from build123d import *

# Parameters (mm, degrees)
SKETCH_1_W          = 10
SKETCH_1_H          = 10
SKETCH_1_W_2        = 8
SKETCH_1_H_2        = 8
EXTRUDE_1_DEPTH     = 50
SKETCH_2_R          = 3
SKETCH_2_R_2        = 1.6
CUT_EXTRUDE_1_DEPTH = 52.961524227
CUT_EXTRUDE_2_REACH = 53.962
SKETCH_4_R          = 2.6
SKETCH_6_R          = 1.6
CUT_EXTRUDE_4_DEPTH = 52.961524227


with BuildPart() as part:
    # ｽｹｯﾁ1 → 押し出し-薄板1 (new body)
    with BuildSketch(Plane.XY):
        with Locations((5, 5)):
            Rectangle(SKETCH_1_W, SKETCH_1_H)
        with Locations((5, 5)):
            Rectangle(SKETCH_1_W_2, SKETCH_1_H_2, mode=Mode.SUBTRACT)
    extrude(amount=EXTRUDE_1_DEPTH)

    # ｽｹｯﾁ2 → ｶｯﾄ - 押し出し1 (cut, through all)
    with BuildSketch(Plane(origin=(0, 10, 0), x_dir=(1, 0, 0), z_dir=(0, 1, 0))):
        with Locations(Location((5, -10.5, 0), (0, 0, 270))):
            Circle(SKETCH_2_R)
        with Locations(Location((5, -19.5, 0), (0, 0, 270))):
            Circle(SKETCH_2_R_2)
        with Locations(Location((5, -34.5, 0), (0, 0, 270))):
            Circle(SKETCH_2_R_2)
    extrude(amount=-CUT_EXTRUDE_1_DEPTH, mode=Mode.SUBTRACT)

    # ｽｹｯﾁ4 → ｶｯﾄ - 押し出し2 (cut, up to next)
    with BuildSketch(Plane.XZ, mode=Mode.PRIVATE) as cut_extrude_2_sk1:
        with Locations(Location((5, 19.5, 0), (0, 0, 270))):
            Circle(SKETCH_4_R)
    cut_extrude_2_tool1 = extrude(cut_extrude_2_sk1.sketch, amount=-CUT_EXTRUDE_2_REACH, mode=Mode.PRIVATE) & part.part
    add(cut_extrude_2_tool1.solids().sort_by_distance((5, 0, 19.5))[0], mode=Mode.SUBTRACT)

    # ｽｹｯﾁ6 → ｶｯﾄ - 押し出し4 (cut, through all)
    with BuildSketch(Plane(origin=(10, 0, 0), x_dir=(0, 0, -1), z_dir=(1, 0, 0))):
        with Locations(Location((-45, 5, 0), (0, 0, 90))):
            Circle(SKETCH_6_R)
    extrude(amount=-CUT_EXTRUDE_4_DEPTH, mode=Mode.SUBTRACT)


solid = part.part
Verification items for the finished model (mm, model axes). A direction names the side the tool comes from. Give positions to 0.01 mm unless a question says otherwise; leave off trailing zeros. Order: outer loops, then holes, each group sorted by start corner. A loop starts at its lowest first (then second) coordinate and runs counter-clockwise, first axis right, second up. Notation, with made-up numbers: M 19,89 L 27,89 A10 ccw 27,105 Z; hole C -31,28.25 d11. An arc over 180 degrees is marked long. Use one line per item in the form item = value. Start each with the question number.
Q1. Section check A-A (y = 2.75). Enter the section's corners in (x, z).
Q2. Section check D-D (z = 37.5). Enter the section's corners in (x, y).
Q3. Mould release check, pull along X, two halves, no side actions. Record for faces 1 (the flat face through (0.5, 5.1, 50)), 2 (the flat face through (10, 5, 25)), 3 (the flat face through (5, 9, 25)): +X half, -X half, draft (parallel to the pull), parting line (faces both ways), or undercut.
Q4. Section check B-B (z = 19.5). Enter the section's corners in (x, y), then the cut area to 3 significant figures.
Q5. Access from +Z, -Z, +X, -X, +Y, -Y to the whole of each face (thin tool, end or side, straight path). Record for faces 4 (the flat face through (5, 0, 25)), 5 (the flat face through (9, 5, 25)), 6 (the cylindrical face through (5.78, 0.49, 17.02)).
Q6. Scan lines: line 1 along X through (y, z) = (3.25, 3.5); line 2 along Z through (x, y) = (9.5, 5). Record each from-to range of solid material in increasing order. Write a range as [from, to].
Q7. Section check C-C (y = 5). Enter the section's corners in (x, z).
Evaluation:
q1.outline = M 0,0 L 1,0 L 1,50 L 0,50 Z; M 9,0 L 10,0 L 10,50 L 9,50 Z
q2.outline = M 0,0 L 10,0 L 10,10 L 0,10 Z; hole M 1,1 L 9,1 L 9,9 L 1,9 Z
q3.face_1 = draft
q3.face_2 = +X half
q3.face_3 = undercut
q4.outline = M 0,0 L 2.4,0 L 2.4,1 L 1,1 L 1,9 L 3.4,9 L 3.4,10 L 0,10 Z; M 6.6,9 L 9,9 L 9,1 L 7.6,1 L 7.6,0 L 10,0 L 10,10 L 6.6,10 Z
q4.area = 27.6 mm2
q5.face_4 = +Z, -Z, +X, -X, -Y
q5.face_5 = +Z, -Z
q5.face_6 = -Y
q6.line_1 = [0, 1], [9, 10]
q6.line_2 = [0, 43.4], [46.6, 50]
q7.outline = M 0,0 L 1,0 L 1,43.4 L 0,43.4 Z; M 0,46.6 L 1,46.6 L 1,50 L 0,50 Z; M 9,0 L 10,0 L 10,43.4 L 9,43.4 Z; M 9,46.6 L 10,46.6 L 10,50 L 9,50 Z
